Autodesk Inventor part; units mm, degrees
ref_plane "YZ Plane" through (0, 0, 0) normal (1, 0, 0) x (0, 1, 0)
ref_plane "XZ Plane" through (0, 0, 0) normal (0, 1, 0) x (-1, 0, 0)
ref_plane "XY Plane" through (0, 0, 0) normal (0, 0, 1) x (1, 0, 0)
sketch "Sketch1" plane through (0, 0, 0) normal (0, 0, 1) x (1, 0, 0)
  circle A0 centre (0.2751, 52.8541) radius 1.4214
  circle A1 centre (53.1386, 52.6394) radius 1.4214
  circle A2 centre (52.924, -0.224) radius 1.4214
  circle A3 centre (0.0605, -0.0094) radius 1.4214
  circle A4 centre (0.2751, 52.8541) radius 1.4214
  circle A5 centre (0.0605, -0.0094) radius 1.4214
  circle A6 centre (52.924, -0.224) radius 1.4214
  circle A7 centre (53.1386, 52.6394) radius 1.4214
  line L0 (-5.2979, -23.5291) -> (88.6821, -23.9107)
  line L1 (88.6821, -23.9107) -> (89.0881, 76.0893)
  line L2 (89.0881, 76.0893) -> (-4.8919, 76.4709)
  line L3 (-4.8919, 76.4709) -> (-5.2979, -23.5291)
  line L4 (-5.2979, -23.5291) -> (2.9514, -23.54) construction
  circle A8 centre (26.5572, 26.3424) radius 11 construction
  circle A9 centre (41.9941, 10.7796) radius 1.5 construction
  circle A10 centre (10.9944, 10.9055) radius 1.5 construction
  circle A11 centre (11.1202, 41.9052) radius 1.5 construction
  circle A12 centre (42.12, 41.7793) radius 1.5 construction
  circle A13 centre (0.2148, 52.8996) radius 1.4224 construction
  circle A14 centre (0, 0) radius 1.4224 construction
  circle A15 centre (52.8996, -0.2148) radius 1.4224 construction
  circle A16 centre (53.1143, 52.6848) radius 1.4224 construction
  line L5 (-5.3215, -5.2784) -> (58.178, -5.5363) construction
  line L6 (58.178, -5.5363) -> (58.4358, 57.9632) construction
  line L7 (58.4358, 57.9632) -> (-5.0637, 58.221) construction
  line L8 (-5.0637, 58.221) -> (-5.3215, -5.2784) construction
  line L9 (88.8851, 26.0893) -> (-5.1926, 26.4713) construction
  line L10 (63.369, -2.4573) -> (63.4464, 16.5925) construction
  line L11 (63.5243, 35.7924) -> (63.6017, 54.8422) construction
  line L12 (63.5243, 35.7924) -> (82.5742, 35.715) construction
  line L13 (63.369, -2.4573) -> (82.4189, -2.5346) construction
  circle A17 centre (71.5076, 7.0347) radius 1.75
  circle A18 centre (71.6629, 45.2844) radius 1.75
  circle A19 centre (71.6629, 45.2844) radius 1.75 construction
  circle A20 centre (71.5076, 7.0347) radius 1.75 construction
  circle A21 centre (72.3353, 26.1565) radius 2.5 construction
  line L14 (65.2233, 18.092) -> (79.4473, 18.092) construction
  line L15 (79.4473, 18.092) -> (79.4473, 34.221) construction
  line L16 (79.4473, 34.221) -> (65.2233, 34.221) construction
  line L17 (65.2233, 34.221) -> (65.2233, 18.092) construction
  line L18 (65.2233, 18.092) -> (79.4473, 34.221) construction
  line L19 (79.4473, 18.092) -> (65.2233, 34.221) construction
  circle A22 centre (79.4473, 18.092) radius 1.4224
  circle A23 centre (65.2233, 18.092) radius 1.4224
  circle A24 centre (79.4473, 34.221) radius 1.4224
  circle A25 centre (65.2233, 34.221) radius 1.4224
  circle A26 centre (79.4473, 18.092) radius 2.6035 construction
  circle A27 centre (65.2233, 18.092) radius 2.6035 construction
  circle A28 centre (79.4473, 34.221) radius 2.6035 construction
  circle A29 centre (65.2233, 34.221) radius 2.6035 construction
  point P0 (0.0605, -0.0094)
  point P1 (88.9156, 66.1637)
  dimension "d7" = 100
  dimension "d8" = 93.98
  dimension "d38" = 3.5
  dimension "d39" = 3.5
  dimension "d40" = 14.224
  dimension "d41" = 16.129
  dimension "d42" = 2.8448
  dimension "d43" = 2.8448
  dimension "d44" = 2.8448
  dimension "d45" = 2.8448
  dimension "d46" = 5.207
  dimension "d47" = 5.207
  dimension "d48" = 5.207
  dimension "d49" = 5.207
extrude "Extrusion1" add sketch "Sketch1" along normal blind 6.35
sketch "Sketch2" plane through (0, 0, 6.35) normal (0, 0, 1) x (1, 0, 0)
  circle A0 centre (0.0605, -0.0094) radius 1.4214 construction
  circle A1 centre (52.924, -0.224) radius 1.4214 construction
  circle A2 centre (53.1386, 52.6394) radius 1.4214 construction
  circle A3 centre (0.2751, 52.8541) radius 1.4214 construction
  line L0 (-5.2979, -23.5291) -> (88.6821, -23.9107) construction
  line L1 (89.0881, 76.0893) -> (-4.8919, 76.4709) construction
  line L2 (-4.8919, 76.4709) -> (-5.2979, -23.5291) construction
  line L3 (89.0881, 76.0893) -> (89.043, 64.9782)
  line L4 (89.043, 64.9782) -> (82.693, 65.004)
  line L5 (82.693, 65.004) -> (82.6479, 53.8929)
  line L6 (82.6479, 53.8929) -> (88.9978, 53.8671)
  line L7 (89.043, 64.9782) -> (88.9978, 53.8671)
  line L8 (88.9979, 53.8673) -> (88.9527, 42.7562)
  line L9 (88.9527, 42.7562) -> (82.6028, 42.782)
  line L10 (82.6028, 42.782) -> (82.5577, 31.6709)
  line L11 (82.5577, 31.6709) -> (88.9076, 31.6451)
  line L12 (88.9527, 42.7562) -> (88.9076, 31.6451)
  line L13 (88.9076, 31.6453) -> (88.8625, 20.5341)
  line L14 (88.8625, 20.5341) -> (82.5126, 20.5599)
  line L15 (82.5126, 20.5599) -> (82.4675, 9.4488)
  line L16 (82.4675, 9.4488) -> (88.8174, 9.423)
  line L17 (88.8625, 20.5341) -> (88.8174, 9.423)
  line L18 (88.8174, 9.4232) -> (88.7723, -1.6879)
  line L19 (88.7723, -1.6879) -> (82.4223, -1.6621)
  line L20 (82.4223, -1.6621) -> (82.3772, -12.7732)
  line L21 (82.3772, -12.7732) -> (88.7272, -12.799)
  line L22 (88.7723, -1.6879) -> (88.7272, -12.799)
  point P0 (0, 0)
  dimension "d12" = 6.35
  dimension "d14" = 11.1111
  dimension "d31" = 22.2222
extrude "Extrusion2" cut sketch "Sketch2" against normal blind 25.4
equation "\"d14\" = d11"
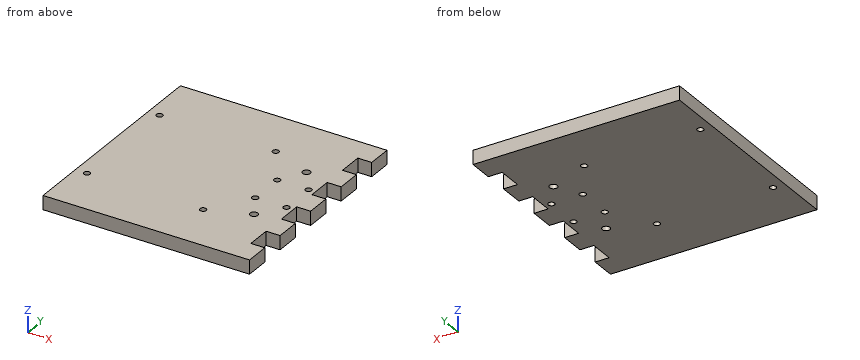
Read the model definition and answer for the solid it produces. Units are mm, in the model's axes. Give positions to 0.01 mm unless a question says otherwise; leave off trailing zeros. Order: outer loops, then holes, each group sorted by start corner. A loop starts at its lowest first (then second) coordinate and runs counter-clockwise, first axis right, second up.
(1) Find section B-B (z = 2.25). Give the number of separate pieces and of enclosed holes in the cut face, plus the area to 3 significant figures.
(2) Find section C-C (y = 15). Give the vertices of the cut face in (x, z).
(3) Find section A-A (x = 71.5). Give the vertices of the cut face in (y, z), plus the area to 3 significant figures.
(4) Straight lines are drawn through the part: L1, parallel to Y at x = 65, z = 1.75; L2, parallel to Y at x = 70.5, z = 2.75; L3, parallel to X at y = 52, z = 1.75. For each, find the intervals that lie inside material, in ascending order.
Result sheet:
1. separate pieces: 1
1. enclosed holes: 10
1. area: 9,050 mm2
2. outline: (-5.14, 0) - (82.49, 0) - (82.49, 6.35) - (-5.14, 6.35) - close
3. outline: (-23.84, 0) - (5.28, 0) - (5.28, 6.35) - (-23.84, 6.35) - close; (8.78, 0) - (43.54, 0) - (43.54, 6.35) - (8.78, 6.35) - close; (47.03, 0) - (76.16, 0) - (76.16, 6.35) - (47.03, 6.35) - close
3. area: 591 mm2
4. L1: y = -23.81 to 16.69, 19.5 to 32.82, 35.63 to 76.19
4. L2: y = -23.84 to 5.6, 8.47 to 43.98, 46.59 to 76.16
4. L3: x = -4.99 to -0.86, 1.41 to 51.87, 54.41 to 88.99
